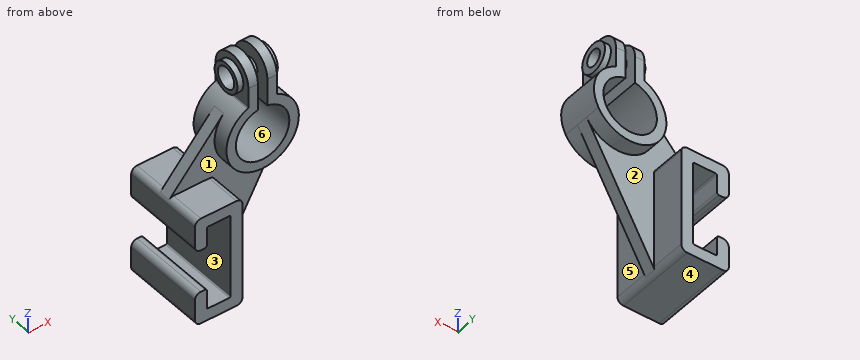
from build123d import *

# Parameters (mm, degrees)
F1_DEPTH  = 18
F2_DEPTH  = 5
F3_DEPTH  = 35
F6_DEPTH  = 8
F8_DEPTH  = 8
F10_DEPTH = 5
F12_DEPTH = 5
F14_D     = 18
F14_DEPTH = 18
F14_TIP   = 5.4077455712
F16_D     = 14
F16_DEPTH = 18
F16_TIP   = 4.2060243332
F17_R     = 1
F18_R     = 1.6
F19_R     = 1


with BuildPart() as f1:
    # F0 (on Front) → F1 (new body, symmetric)
    with BuildSketch(Plane.XZ):
        with BuildLine():
            ThreePointArc((4, 22.1415898255), (0, -22.5), (-4, 22.1415898255))
            Line((-4, 22.1415898255), (-4, 45))
            Line((-4, 45), (-12, 45))
            Line((-12, 45), (-12, 28.0401497856))
            ThreePointArc((-12, 28.0401497856), (-17.8577847603, 24.7254832805), (-22.845943753, 20.2067526841))
            ThreePointArc((-22.845943753, 20.2067526841), (-17.587930353, -24.9181601628), (26.691644965, -14.7582549463))
            ThreePointArc((26.691644965, -14.7582549463), (28.8476465145, 9.9026910774), (12, 28.0401497856))
            Line((12, 28.0401497856), (12, 45))
            Line((12, 45), (4, 45))
            Line((4, 45), (4, 22.1415898255))
        make_face()
    extrude(amount=F1_DEPTH, both=True)

    # F0 (on Front) → F2 (join, symmetric)
    with BuildSketch(Plane.XZ):
        with BuildLine():
            ThreePointArc((26.691644965, -14.7582549463), (-17.587930353, -24.9181601628), (-22.845943753, 20.2067526841))
            Line((-22.845943753, 20.2067526841), (-68.7452366808, -31.6874175928))
            ThreePointArc((-68.7452366808, -31.6874175928), (-67.0539094386, -30.4413317714), (-65, -30))
            Line((-65, -30), (-35, -30))
            ThreePointArc((-35, -30), (-31.4644660941, -31.4644660941), (-30, -35))
            Line((-30, -35), (-30, -116))
            ThreePointArc((-30, -116), (-30.1585953736, -117.2493203127), (-30.6243204975, -118.4193860568))
            Line((-30.6243204975, -118.4193860568), (26.691644965, -14.7582549463))
        make_face()
    extrude(amount=F2_DEPTH, both=True)

    # F0 (on Front) → F3 (join, symmetric)
    with BuildSketch(Plane.XZ):
        with BuildLine():
            ThreePointArc((-65, -30), (-67.0539094386, -30.4413317714), (-68.7452366808, -31.6874175928))
            ThreePointArc((-68.7452366808, -31.6874175928), (-69.6757985096, -33.2288680744), (-70, -35))
            Line((-70, -35), (-70, -52.5))
            ThreePointArc((-70, -52.5), (-68.5355339059, -56.0355339059), (-65, -57.5))
            Line((-65, -57.5), (-60, -57.5))
            Line((-60, -57.5), (-60, -40))
            Line((-60, -40), (-40, -40))
            Line((-40, -40), (-40, -111))
            Line((-40, -111), (-60, -111))
            Line((-60, -111), (-60, -93.5))
            Line((-60, -93.5), (-65, -93.5))
            ThreePointArc((-65, -93.5), (-68.5355339059, -94.9644660941), (-70, -98.5))
            Line((-70, -98.5), (-70, -116))
            ThreePointArc((-70, -116), (-68.5355339059, -119.5355339059), (-65, -121))
            Line((-65, -121), (-35, -121))
            ThreePointArc((-35, -121), (-32.4600128232, -120.3067929068), (-30.6243204975, -118.4193860568))
            ThreePointArc((-30.6243204975, -118.4193860568), (-30.1585953736, -117.2493203127), (-30, -116))
            Line((-30, -116), (-30, -35))
            ThreePointArc((-30, -35), (-31.4644660941, -31.4644660941), (-35, -30))
            Line((-35, -30), (-65, -30))
        make_face()
    extrude(amount=F3_DEPTH, both=True)

    # F5 (on face) → F6 (join, through all)
    with BuildSketch(Plane.YZ.offset(12)):
        with BuildLine():
            Line((-18, 45), (18, 45))
            ThreePointArc((18, 45), (0, 63), (-18, 45))
        make_face()
    extrude(amount=-F6_DEPTH)

    # F7 (on face) → F8 (join, through all)
    with BuildSketch(Plane(origin=(-12, 0, 0), x_dir=(0, -1, 0), z_dir=(-1, 0, 0))):
        with BuildLine():
            Line((-18, 45), (18, 45))
            ThreePointArc((18, 45), (0, 63), (-18, 45))
        make_face()
    extrude(amount=-F8_DEPTH)

    # F9 (on face) → F10 (join)
    with BuildSketch(Plane(origin=(-12, 0, 0), x_dir=(0, -1, 0), z_dir=(-1, 0, 0))):
        with BuildLine():
            Line((-12.5, 45), (12.5, 45))
            ThreePointArc((12.5, 45), (0, 57.5), (-12.5, 45))
        make_face()
        with BuildLine():
            ThreePointArc((-12.5, 45), (0, 32.5), (12.5, 45))
            Line((12.5, 45), (-12.5, 45))
        make_face()
    extrude(amount=F10_DEPTH)

    # F11 (on face) → F12 (join)
    with BuildSketch(Plane.YZ.offset(12)):
        with BuildLine():
            Line((-12.5, 45), (12.5, 45))
            ThreePointArc((12.5, 45), (0, 57.5), (-12.5, 45))
        make_face()
        with BuildLine():
            ThreePointArc((-12.5, 45), (0, 32.5), (12.5, 45))
            Line((12.5, 45), (-12.5, 45))
        make_face()
    extrude(amount=F12_DEPTH)

    # F14
    with Locations(Plane(origin=(-17, 0, 0), x_dir=(0, -1, 0), z_dir=(-1, 0, 0))):
        with Locations((0, 45)):
            Hole(F14_D / 2, depth=F14_DEPTH)
            with Locations((0, 0, -(F14_DEPTH + F14_TIP / 2))):  # 118° drill point
                Cone(0, F14_D / 2, F14_TIP, mode=Mode.SUBTRACT)

    # F16
    with Locations(Plane.YZ.offset(17)):
        with Locations((0, 45)):
            Hole(F16_D / 2, depth=F16_DEPTH)
            with Locations((0, 0, -(F16_DEPTH + F16_TIP / 2))):  # 118° drill point
                Cone(0, F16_D / 2, F16_TIP, mode=Mode.SUBTRACT)

    # F17
    f17_edges = [f1.edges().sort_by_distance(p)[0] for p in [
        (-60, 0, -40),
        (-40, 0, -40),
        (-40, 0, -111),
        (-60, 0, -111),
    ]]
    fillet(f17_edges, radius=F17_R)

    # F18
    f18_edges = [f1.edges().sort_by_distance(p)[0] for p in [
        (-60, 0, -57.5),
        (-60, 0, -93.5),
    ]]
    fillet(f18_edges, radius=F18_R)

    # F19
    f19_edges = [f1.edges().sort_by_distance(p)[0] for p in [
        (12, 9, 28.04015),
        (12, -9, 28.04015),
        (-12, 9, 28.04015),
        (-12, -9, 28.04015),
    ]]
    fillet(f19_edges, radius=F19_R)


solid = f1.part
Could you check a few things on this model? Use its own coordinates, in mm. Face numbers are marked on the shaded views. A direction names the side the tool comes from. Round coordinates to 2 decimals unless told otherwise and drop trailing zeros. Write each loop counter-clockwise with the first axis right and the second up, starting at its lowest first coordinate (ties: lowest second). Pieces come first, ordered by that corner, then holes. Notation, with made-up numbers: (24, -38) - (62, -38) arc R36 ccw to (62, -3) - close; hole circle Ø6 at (74, 70). An arc over 180 degrees is marked (long way). Put each result on its own line as item: value. Start each with the question number.
(1) I want a section at A-A, the plane y = 0. Give the number of separate pieces and of enclosed holes in the cut face, plus the area to 3 significant figures.
(2) I want a section at B-B, the plane x = -54.5. Please give me the cut outline in (y, z).
(3) Thinking about a two-plate mould opening in X: for the marked faces 4, 5 and 6, which applies, released by +X, released by -X, zero draft, split by the parting line, or undercut?
(4) I want a section at D-D, the plane y = 27. Please give me the cut outline in (x, z), plus the area to 3 significant figures.
(5) For the marked faces 1, 2 and 3, which set-ups out of +Z, -Z, +X, -X, +Y, -Y let a thin tool reach every point of the face, with its end or its side?
(6) Will these pins go through, and if not, where does the flat tip stop? pin 1 (8.5 mm diameter, centred on y = 0, z = 45, fed in from +X); pin 2 (24 mm diameter, centred on y = -17.5, z = -86, fed in from +X); pin 3 (10 mm diameter, centred on x = 13.5, y = 15.5, fed in from +Z); pin 4 (24 mm diameter, centred on x = -52, y = 18, fed in from +Z).
(7) I want a section at C-C, the plane z = 0. Please give me the cut outline in (x, y), plus the area to 3 significant figures.
(8) I need wall thicknesses on probe 1 along X at (y, z) = (-29.5, -103); probe 2 along Z at (x, y) = (-55, 12); probe 3 along X at (y, z) = (12, 54.5). Which ranges of each line are inside material? Lowest first, please.
Here are the results:
1. separate pieces: 3
1. enclosed holes: 0
1. area: 6,590 mm^2
2. outline: (-35, -121) - (35, -121) - (35, -111) - (-35, -111) - close; (-35, -40) - (35, -40) - (35, -30) - (5, -30) - (5, -15.58) - (-5, -15.58) - (-5, -30) - (-35, -30) - close
3. face 4: zero draft
3. face 5: released by +X
3. face 6: undercut
4. outline: (-70, -116) arc R5 ccw to (-65, -121) - (-35, -121) arc R5 ccw to (-30, -116) - (-30, -35) arc R5 ccw to (-35, -30) - (-65, -30) arc R5 ccw to (-70, -35) - (-70, -52.5) arc R5 ccw to (-65, -57.5) - (-61.6, -57.5) arc R1.6 ccw to (-60, -55.9) - (-60, -41) arc R1 cw to (-59, -40) - (-41, -40) arc R1 cw to (-40, -41) - (-40, -110) arc R1 cw to (-41, -111) - (-59, -111) arc R1 cw to (-60, -110) - (-60, -95.1) arc R1.6 ccw to (-61.6, -93.5) - (-65, -93.5) arc R5 ccw to (-70, -98.5) - close
4. area: 1,830 mm^2
5. face 1: -Y
5. face 2: +Y
5. face 3: +Y, -Y
6. pin 1: passes through
6. pin 2: stops at x = -30
6. pin 3: stops at z = 59.45
6. pin 4: stops at z = -30
7. outline: (-40.72, -5) - (-30.5, -5) - (-30.5, -18) - (-22.5, -18) - (-22.5, 18) - (-30.5, 18) - (-30.5, 5) - (-40.72, 5) - close; (22.5, -18) - (30.5, -18) - (30.5, 18) - (22.5, 18) - close
7. area: 678 mm^2
8. probe 1: x = -70 to -60, -40 to -30
8. probe 2: z = -121 to -111, -40 to -30
8. probe 3: x = -12 to -4, 4 to 12
